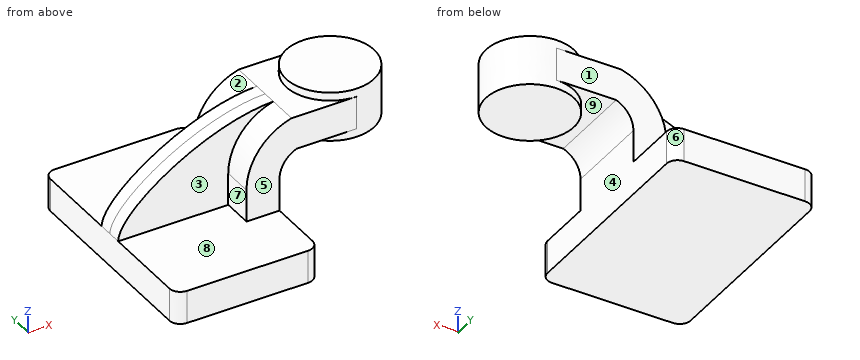
```python
from build123d import *

# Parameters (mm, degrees)
F1_DEPTH = 25.4
F2_DEPTH = 63.5
F3_DEPTH = 7.9375
F5_R     = 6.35


with BuildPart() as f1:
    # F0 (on Front) → F1 (new body, symmetric)
    with BuildSketch(Plane.XZ):
        with BuildLine():
            Line((22.225, 28.1521443485), (22.225, 9.525))
            Line((22.225, 9.525), (41.275, 9.525))
            Line((41.275, 9.525), (41.275, 28.1521443485))
            ThreePointArc((41.275, 28.1521443485), (43.992026211, 37.0337743098), (51.2130599394, 42.8752))
            Line((51.2130599394, 42.8752), (60.325, 42.8752))
            Line((60.325, 42.8752), (60.325, 61.9252))
            Line((60.325, 61.9252), (48.2541393355, 61.9252))
            ThreePointArc((48.2541393355, 61.9252), (29.4873576939, 49.4719437295), (22.225, 28.1521443485))
        make_face()
        Polygon((85.7263787281, 61.9252), (60.325, 61.9252), (60.325, 42.8752), (85.7319083861, 42.8752), align=None)
    extrude(amount=F1_DEPTH, both=True)

    # F0 (on Front) → F2 (join, symmetric)
    with BuildSketch(Plane.XZ):
        Polygon((22.225, 9.525), (-41.275, 9.525), (-41.275, -9.525), (41.275, -9.525), (41.275, 9.525), align=None)
    extrude(amount=F2_DEPTH, both=True)

    # F0 (on Front) → F3 (join, symmetric)
    with BuildSketch(Plane.XZ):
        with BuildLine():
            add(Edge.make_bspline(
                [(-41.275, 9.525), (-40.7644435763, 26.8716271967), (9.3228099868, 60.8724653721), (48.2541393355, 61.9252)],
                knots=[0, 0, 0, 0, 103.7364340538, 103.7364340538, 103.7364340538, 103.7364340538], degree=3))
            Line((-41.275, 9.525), (22.225, 9.525))
            Line((22.225, 9.525), (22.225, 28.1521443485))
            ThreePointArc((22.225, 28.1521443485), (29.4873576939, 49.4719437295), (48.2541393355, 61.9252))
        make_face()
    extrude(amount=F3_DEPTH, both=True)

    # F0 (on Front) → F4 (revolve)
    with BuildSketch(Plane.XZ):
        Polygon((85.725, 66.675), (85.7263787281, 61.9252), (85.7319083861, 42.8752), (85.733294487, 38.1), (111.125, 38.1), (111.125, 66.675), align=None)
    revolve(axis=Axis((85.7291472435, 0, 52.3875), (0.0002902707, 0, -0.9999999579)))

    # F5
    f5_edges = [f1.edges().sort_by_distance(p)[0] for p in [
        (-41.275, -63.5, 0),
        (41.275, -63.5, 0),
        (-41.275, 63.5, 0),
        (41.275, 63.5, 0),
    ]]
    fillet(f5_edges, radius=F5_R)


solid = f1.part
```
The listing builds one solid part. Answer for the finished solid, in the listing's coordinates (mm). Face numbers are marked on the shaded views. A direction names the side the tool comes from. Coordinates: 2 decimals unless noted, no trailing zeros. Loops run counter-clockwise (first coordinate to the right, second up) from the corner with the lowest first, then second, coordinate; pieces in that order, holes last. Notation, with made-up numbers: (-17, 74.5) -> (-9, 74.5) arc R8 ccw to (-9, 88.5) -> close; hole circle Ø10 at (76, -23.5). An arc over 180 degrees is marked (long way). Use one line per item in the form item = value. Start each with the question number.
Item 1: The mould has two halves that part along X. Classify the marked faces 6, 7, 8 and 9: released by +X, released by -X, zero draft, split by the parting line, or undercut.
Item 2: A tool of negligible diameter and unlimited length cuts with its end or side. For the marked faces 1, 2, 3, 4 and 5, from which of +Z, -Z, +X, -X, +Y, -Y can it reach the whole face along a straight path? Write none if from no direction.
Item 3: Consider L1, parallel to Y at x = 28.5, z = 41; L2, parallel to Z at x = 24, y = -50.5 (3 decimals); L3, parallel to Z at x = 98.5, y = -15.5. Determine where each line is inside the solid, lowest interval first. Write a range as [from, to].
Item 4: Flat-ended cylindrical pins translate along their axes: pin 1 Ø16.5 at (x, y) = (4, -44.5) entering from +Z (3 decimals); pin 2 Ø19 at (y, z) = (-20, 1.5) entering from +X (3 decimals); pin 3 Ø14 at (y, z) = (15.5, 20) entering from -X (3 decimals). Find the tip coordinate at first contact, or state that the pin passes through.
Item 5: The part is cut by section A-A on z = -1. Determine the outline of the cut face in (x, y) (3 decimals).
Item 6: The part is cut by section C-C on x = 56. Determine the outline of the cut face in (y, z).
Item 7: The part is cut by section B-B on y = 52. Determine the outline of the cut face in (x, z) (3 decimals), then the cut area to 3 significant figures.
Answer key:
q1.face_6 = released by +X
q1.face_7 = released by -X
q1.face_8 = zero draft
q1.face_9 = undercut
q2.face_1 = +Z, +X, -X, +Y
q2.face_2 = +Z, -X, +Y
q2.face_3 = +Z, -X, -Y
q2.face_4 = -Z, +X, +Y, -Y
q2.face_5 = +Z, +X, -X, -Y
q3.L1 = [-25.4, 25.4]
q3.L2 = [-9.525, 9.525]
q3.L3 = [38.1, 66.67]
q4.pin_1 = 9.525
q4.pin_2 = 41.275
q4.pin_3 = 22.225
q5.outline = (-41.275, -57.15) arc R6.35 ccw to (-34.925, -63.5) -> (34.925, -63.5) arc R6.35 ccw to (41.275, -57.15) -> (41.275, 57.15) arc R6.35 ccw to (34.925, 63.5) -> (-34.925, 63.5) arc R6.35 ccw to (-41.275, 57.15) -> close
q6.outline = (-25.4, 42.88) -> (25.4, 42.88) -> (25.4, 61.93) -> (-25.4, 61.93) -> close
q7.outline = (-41.275, -9.525) -> (41.275, -9.525) -> (41.275, 9.525) -> (-41.275, 9.525) -> close
q7.area = 1,570 mm2
